from build123d import *

# Parameters (mm, degrees)
F1_DEPTH = 3.03784
F2_R     = 2.38125
F3_DEPTH = 3.03784
F4_R     = 1.5875
F5_R     = 1.51882


# Not quite as in the source:
# - a fillet or chamfer is up to 0.001 mm smaller than in the source, because OpenCascade refuses the exact size


with BuildPart() as f1:
    # F0 (on Front) → F1 (new body)
    with BuildSketch(Plane.XZ):
        with BuildLine():
            Line((-65.2018, 74.2696), (-65.2018, -19.7612))
            add(Edge.make_bspline(
                [(-65.2018, -19.7612), (-60.7850037253, -18.6171418479), (-51.9575306305, -16.3306106319), (-38.8253253798, -12.61749568), (-25.7966517502, -8.6478861048), (-12.8391741047, -4.4585465011), (0.0137529583, -0.0438991729), (12.7925184797, 4.6371253852), (25.4667360287, 9.5345524455), (38.0928063194, 14.6983578431), (50.6196821862, 20.0682362577), (58.915858645, 23.8585166667), (63.0682, 25.7556)],
                knots=[0, 0, 0, 0, 0.1001945647, 0.2002503103, 0.3002105802, 0.4001552007, 0.5000116128, 0.5999162071, 0.6997672128, 0.7997893994, 0.8997920596, 1, 1, 1, 1], degree=3))
            Line((63.0682, 25.7556), (63.0682, 74.2696))
            Line((63.0682, 74.2696), (-65.2018, 74.2696))
        make_face()
    extrude(amount=F1_DEPTH)

    # F2 (on face) → F3 (cut, through all)
    with BuildSketch(Plane.XZ.offset(3.03784)):
        with Locations((-60.4393, 64.7446)):
            Circle(F2_R)
        with Locations((-60.4393, 26.6446)):
            Circle(F2_R)
        with Locations((-12.8143, 64.7446)):
            Circle(F2_R)
        with Locations((37.9857, 64.7446)):
            Circle(F2_R)
    extrude(amount=-F3_DEPTH, mode=Mode.SUBTRACT)

    # F4
    f4_edges = [f1.edges().sort_by_distance(p)[0] for p in [
        (-65.2018, -1.51892, 74.2696),
        (63.0682, -1.51892, 74.2696),
    ]]
    fillet(f4_edges, radius=F4_R)

    # F5 (radius 1.51892 in the source; OpenCascade refuses exactly that, so slightly less here)
    f5_edges = [f1.edges().sort_by_distance(p)[0] for p in [
        (-0.002981, -3.03784, -0.001058),
        (-0.002981, 0, -0.001058),
    ]]
    fillet(f5_edges, radius=F5_R)


solid = f1.part
Build history of the part. All positions in model axes, mm. Round coordinates to 2 decimals unless told otherwise and drop trailing zeros. Use CSV: the item, a comma, the result in double quotes. Start each with the question number.
Q1. Mould opens along X. For faces 1 (the face through (-13.33, -1.54, 62.42)), 2 (the face through (-65.202, -1, 27)), 3 (the face through (-2, 0, 39)), 4 (the face through (-60.96, -1.54, 62.42)) say: +X half, -X half, draft (parallel to the pull), parting line (faces both ways), or undercut.
Q2. Drill centre lines: L1, parallel to Z at x = -11.5, y = -2.7; L2, parallel to Z at x = -13, y = -0.75; L3, parallel to Z at x = 51, y = -1.65. Where is each one in solid material? Low to high.
Q3. Saw through at A-A on y = -2.5. Count the separate pieces of the cut face and the enclosed holes in it, and give its area (3 significant figures).
Q4. Flat gauge pin, fed straight in: pin 1 Ø12 at (x, z) = (40, 9.5) entering from -Y. Where does the tip first touch, or does it go through?
Solutions:
1,face 1,"undercut"
1,face 2,"-X half"
1,face 3,"draft"
1,face 4,"undercut"
2,L1,"z = -3.37 to 62.76, 66.73 to 74.27"
2,L2,"z = -4.25 to 62.37, 67.12 to 74.27"
2,L3,"z = 20.3 to 74.27"
3,separate pieces,"1"
3,enclosed holes,"4"
3,area,"9,310 mm^2"
4,pin 1,"stops at y = -2.58"
